from build123d import *

# Parameters (mm, degrees)
SKETCH6_W            = 105
SKETCH6_H            = 83
BOSS_EXTRUDE3_DEPTH  = 4.5
SKETCH9_W            = 3
SKETCH9_H            = 101
CUT_EXTRUDE6_DEPTH   = 81
SKETCH10_W           = 1
SKETCH10_H           = 8
BOSS_EXTRUDE4_DEPTH  = 8
SKETCH11_W           = 1.226225524
SKETCH11_H           = 5
BOSS_EXTRUDE5_DEPTH  = 5
BOSS_EXTRUDE12_DEPTH = 1.226226
SKETCH27_W           = 15
SKETCH27_H           = 2
SKETCH27_W_2         = 41
SKETCH27_W_3         = 11
SKETCH27_H_2         = 15
BOSS_EXTRUDE20_DEPTH = 30
SKETCH28_W           = 1.5
SKETCH28_H           = 11
BOSS_EXTRUDE21_DEPTH = 3
SKETCH29_W           = 41
SKETCH29_H           = 2
BOSS_EXTRUDE22_DEPTH = 30
SKETCH30_W           = 2
SKETCH30_H           = 38
BOSS_EXTRUDE23_DEPTH = 60
SKETCH31_R           = 5
BOSS_EXTRUDE24_DEPTH = 35
DRAFT1_ANGLE         = -3.5
DRAFT3_ANGLE         = -3.5
SKETCH32_W           = 4
SKETCH32_H           = 28
BOSS_EXTRUDE25_DEPTH = 7
SKETCH33_W           = 4
SKETCH33_H           = 26
BOSS_EXTRUDE26_DEPTH = 5
SKETCH39_W           = 41
SKETCH39_H           = 24
BOSS_EXTRUDE30_DEPTH = 2
SKETCH40_R           = 5
CUT_EXTRUDE9_DEPTH   = 2
BOSS_EXTRUDE31_DEPTH = 15
SKETCH42_W           = 15
SKETCH42_H           = 2
BOSS_EXTRUDE32_DEPTH = 4
SKETCH45_W           = 30
SKETCH45_H           = 18
CUT_EXTRUDE10_DEPTH  = 5
FILLET1_R            = 4
FILLET2_R            = 4


with BuildPart() as part:
    # Sketch6 → Boss-Extrude3 (new body)
    with BuildSketch(Plane(origin=(0, 0, 0), x_dir=(0, 0, -1), z_dir=(1, 0, 0))):
        with Locations((52.5, -41.5)):
            Rectangle(SKETCH6_W, SKETCH6_H)
    extrude(amount=BOSS_EXTRUDE3_DEPTH)

    # Sketch9 → Cut-Extrude6 (cut)
    with BuildSketch(Plane.XZ.offset(83)):
        with Locations((3, -52.5)):
            Rectangle(SKETCH9_W, SKETCH9_H)
    extrude(amount=-CUT_EXTRUDE6_DEPTH, mode=Mode.SUBTRACT)

    # Sketch10 → Boss-Extrude4 (add)
    with BuildSketch(Plane(origin=(0, 0, -2), x_dir=(-1, 0, 0), z_dir=(0, 0, -1))):
        with Locations((-4, -6)):
            Rectangle(SKETCH10_W, SKETCH10_H)
    extrude(amount=BOSS_EXTRUDE4_DEPTH)

    # Sketch11 → Boss-Extrude5 (add)
    with BuildSketch(Plane.XY.offset(-103)):
        with Locations((3.886887238, -4.5)):
            Rectangle(SKETCH11_W, SKETCH11_H)
    extrude(amount=BOSS_EXTRUDE5_DEPTH)

    # Sketch18 → Boss-Extrude12 (add)
    with BuildSketch(Plane(origin=(4.5, 0, 0), x_dir=(0, 0, -1), z_dir=(1, 0, 0))):
        Polygon((103, -12), (93, -2), (103, -2), align=None)
        Polygon((18, -2), (2, -2), (2, -18), align=None)
    extrude(amount=-BOSS_EXTRUDE12_DEPTH)

    # Sketch27 → Boss-Extrude20 (add)
    with BuildSketch(Plane.ZY):
        with Locations((-112.5, -54)):
            Rectangle(SKETCH27_W, SKETCH27_H)
        with Locations((-125.5, -19)):
            Rectangle(SKETCH27_W_2, SKETCH27_H)
        with Locations((-110.5, -1.5)):
            Rectangle(SKETCH27_W_3, SKETCH27_H_2)
        with Locations((-140.5, -1.5)):
            Rectangle(SKETCH27_W_3, SKETCH27_H_2)
    extrude(amount=-BOSS_EXTRUDE20_DEPTH)


with BuildPart() as boss_extrude20_piece_1:
    # of the separate pieces the step leaves, piece 1, a body of its own (boss_extrude20_pieces)
    add(part.part.solids().sort_by_distance((0, 0, 0))[0])



with BuildPart() as boss_extrude20_piece_2:
    # of the separate pieces the step leaves, piece 2, a body of its own (boss_extrude20_pieces)
    add(part.part.solids().sort_by_distance((0, 6, -146))[0])


with BuildPart() as boss_extrude20_piece_1_1:
    add(boss_extrude20_piece_1.part)

    add(boss_extrude20_piece_2.part)  # Boss-Extrude21 merges Boss-Extrude20 piece 2
    # Sketch28 → Boss-Extrude21 (add)
    with BuildSketch(Plane(origin=(30, 0, 0), x_dir=(0, 0, -1), z_dir=(1, 0, 0))):
        with Locations((145.25, -14.5)):
            Rectangle(SKETCH28_W, SKETCH28_H)
        with Locations((105.75, -14.5)):
            Rectangle(SKETCH28_W, SKETCH28_H)
    extrude(amount=-BOSS_EXTRUDE21_DEPTH)

    # Sketch29 → Boss-Extrude22 (add)
    with BuildSketch(Plane(origin=(30, 0, 0), x_dir=(0, 0, -1), z_dir=(1, 0, 0))):
        with Locations((125.5, 5)):
            Rectangle(SKETCH29_W, SKETCH29_H)
    extrude(amount=-BOSS_EXTRUDE22_DEPTH)

    # Sketch30 → Boss-Extrude23 (add)
    with BuildSketch(Plane(origin=(0, 0, -105), x_dir=(-1, 0, 0), z_dir=(0, 0, -1))):
        with Locations((-1, -39)):
            Rectangle(SKETCH30_W, SKETCH30_H)
    extrude(amount=BOSS_EXTRUDE23_DEPTH)

    # Sketch31 → Boss-Extrude24 (add)
    with BuildSketch(Plane(origin=(2, 0, 0), x_dir=(0, 0, -1), z_dir=(1, 0, 0))):
        with Locations(Location((159, -52, 0), (0, 0, 180))):
            Circle(SKETCH31_R)
        with Locations(Location((159, -26, 0), (0, 0, 180))):
            Circle(SKETCH31_R)
    extrude(amount=BOSS_EXTRUDE24_DEPTH)

    # Draft1
    draft1_faces = [boss_extrude20_piece_1_1.faces().sort_by_distance(p)[0] for p in [
        (19.5, -52, -164),
    ]]
    draft(draft1_faces, Plane(origin=(37, -52, -159), x_dir=(0, 0, 1), z_dir=(1, 0, 0)), DRAFT1_ANGLE)

    # Draft3
    draft3_faces = [boss_extrude20_piece_1_1.faces().sort_by_distance(p)[0] for p in [
        (19.5, -26, -164),
    ]]
    draft(draft3_faces, Plane(origin=(37, -26, -159), x_dir=(0, 0, 1), z_dir=(1, 0, 0)), DRAFT3_ANGLE)

    # Sketch32 → Boss-Extrude25 (add)
    with BuildSketch(Plane(origin=(2, 0, 0), x_dir=(0, 0, -1), z_dir=(1, 0, 0))):
        with Locations((159, -39)):
            Rectangle(SKETCH32_W, SKETCH32_H)
    extrude(amount=BOSS_EXTRUDE25_DEPTH)

    # Sketch33 → Boss-Extrude26 (add)
    with BuildSketch(Plane(origin=(37, 0, 0), x_dir=(0, 0, -1), z_dir=(1, 0, 0))):
        with Locations((159, -39)):
            Rectangle(SKETCH33_W, SKETCH33_H)
    extrude(amount=-BOSS_EXTRUDE26_DEPTH)

    # Sketch39 → Boss-Extrude30 (add)
    with BuildSketch(Plane.ZY):
        with Locations((-125.5, -6)):
            Rectangle(SKETCH39_W, SKETCH39_H)
    extrude(amount=-BOSS_EXTRUDE30_DEPTH)

    # Sketch40 → Cut-Extrude9 (cut)
    with BuildSketch(Plane(origin=(2, 0, 0), x_dir=(0, 0, -1), z_dir=(1, 0, 0))):
        with Locations((125.5, -6.5)):
            Circle(SKETCH40_R)
    extrude(amount=-CUT_EXTRUDE9_DEPTH, mode=Mode.SUBTRACT)

    # Sketch41 → Boss-Extrude31 (add)
    with BuildSketch(Plane(origin=(0, 0, -120), x_dir=(-1, 0, 0), z_dir=(0, 0, -1))):
        Polygon((-2, -55), (-2, -58), (-4.5, -55), align=None)
        Polygon((-2, -50), (-4.5, -53), (-2, -53), align=None)
    extrude(amount=-BOSS_EXTRUDE31_DEPTH)

    # Sketch42 → Boss-Extrude32 (add)
    with BuildSketch(Plane(origin=(30, 0, 0), x_dir=(0, 0, -1), z_dir=(1, 0, 0))):
        with Locations((112.5, -54)):
            Rectangle(SKETCH42_W, SKETCH42_H)
    extrude(amount=BOSS_EXTRUDE32_DEPTH)

    # Sketch45 → Cut-Extrude10 (cut)
    with BuildSketch(Plane(origin=(2, 0, 0), x_dir=(0, 0, -1), z_dir=(1, 0, 0))):
        with Locations((120, -29)):
            Rectangle(SKETCH45_W, SKETCH45_H)
    extrude(amount=-CUT_EXTRUDE10_DEPTH, mode=Mode.SUBTRACT)

    # Fillet1
    fillet1_edges = [boss_extrude20_piece_1_1.edges().sort_by_distance(p)[0] for p in [
        (15, 6, -146),
    ]]
    fillet(fillet1_edges, radius=FILLET1_R)

    # Fillet2
    fillet2_edges = [boss_extrude20_piece_1_1.edges().sort_by_distance(p)[0] for p in [
        (15, 6, -105),
    ]]
    fillet(fillet2_edges, radius=FILLET2_R)


solid = boss_extrude20_piece_1_1.part
The listing builds one solid part. Answer for the finished solid, in the listing's coordinates (mm). A direction names the side the tool comes from. Give positions to 0.01 mm unless a question says otherwise; leave off trailing zeros. Order: outer loops, then holes, each group sorted by start corner. A loop starts at its lowest first (then second) coordinate and runs counter-clockwise, first axis right, second up. Notation, with made-up numbers: (19, -4.5) - (27, -4.5) arc R25 cw to (27, 31.5) - close; hole circle Ø7 at (-3.5, 74.25). An arc over 180 degrees is marked (long way). One line per item, written item: value. Start each with the question number.
1) Find the intervals of material crossed by L1, parallel to Y at x = 1.25, z = -125.5; L2, parallel to Y at x = 12, z = -119.5; L3, parallel to Z at x = 15, y = -0.5, in increasing order.
2) A cutting plane is placed at C-C on z = -159. Give the vertices of the cut face in (x, y), then the cut area to 3 significant figures.
3) A tool of negligible diameter and unlimited length cuts with its end or side. For faces 4 (the face through (19, -53, -112)), 5 (the face through (3.232, -51.479, -112.605)), 6 (the face through (19.26, -22.18, -159.85)), from which of +Z, -Z, +X, -X, +Y, -Y can it reach the whole face along a straight path? Write none if from no direction.
4) A cutting plane is placed at D-D on y = -73.5. Give the vertices of the cut face in (x, z).
5) A cutting plane is placed at A-A on z = -125.5. Give the vertices of the cut face in (x, y).
6) Given pin 1 Ø1.5 at (x, y) = (33.5, -34.5) entering from +Z; pin 2 Ø1 at (x, z) = (1, -146.5) entering from -Y; pin 3 Ø7.5 at (x, z) = (22.5, -111) entering from -Y, each flat-ended and moving along its own axis, determine where each tip first touches the part or whether it passes through.
7) The mould has two halves that part along Z. Classify faces 1 (the face through (15.21, 4.859, -106.203)), 2 (the face through (3, -33, -105)), 3 (the face through (4.5, -1, -64)): released by +Z, released by -Z, zero draft, split by the parting line, or undercut.
8) A cutting plane is placed at B-B on y = -26. Give the vertices of the cut face in (x, z), then the cut area to 3 significant figures.
Answer sheet:
1. L1: y = -58 to -38, -20 to -11.5, -1.5 to 6
1. L2: y = -55 to -53, -20 to -18, 4 to 6
1. L3: z = -146 to -135, -116 to -105
2. outline: (0, -58) - (2, -58) - (2, -54.86) - (37, -57) - (37, -21) - (2, -23.14) - (2, -20) - (0, -20) - close; hole (9, -48.71) - (32, -47.31) - (32, -30.69) - (9, -29.29) - close
2. area: 847 mm2
3. face 4: +Z, +X
3. face 5: +X
3. face 6: none
4. outline: (0, -105) - (4.5, -105) - (4.5, -103) - (1.5, -103) - (1.5, -2) - (4.5, -2) - (4.5, 0) - (0, 0) - close
5. outline: (0, -58) - (2, -58) - (2, -38) - (0, -38) - close; (0, -20) - (30, -20) - (30, -18) - (2, -18) - (2, -11.5) - (0, -11.5) - close; (0, -1.5) - (2, -1.5) - (2, 4) - (30, 4) - (30, 6) - (0, 6) - close
6. pin 1: stops at z = -157
6. pin 2: stops at y = -58
6. pin 3: stops at y = -55
7. face 1: released by +Z
7. face 2: undercut
7. face 3: zero draft
8. outline: (0, -165) - (2, -165) - (2, -161.86) - (37, -164) - (37, -154) - (2, -156.14) - (2, -135) - (0, -135) - close; (0, -105) - (4.5, -105) - (4.5, -103) - (1.5, -103) - (1.5, -2) - (4.5, -2) - (4.5, 0) - (0, 0) - close
8. area: 505 mm2
